Answer from the drawing. Dimensions are ordinates in mm from the lowest x, y and z of the part. Coordinates: 2 decimals unless noted, no trailing zeros. Order: outer loops, then holes, each group sorted by start corner. A loop starts at its lowest first (then second) coordinate and runs counter-clockwise, first axis right, second up. Notation, with made-up numbers: (-20, -7.75) -> (30, -7.75) arc R35 cw to (30, 31.25) -> close; hole circle Ø9 at (-14.5, 66). An arc over 180 degrees is marked (long way). Answer as a JSON object with one key per item and string values. Group by question number.
1) Consider L1, parallel to Y at x = 1.9, z = 10.5; L2, parallel to Y at x = 1.1, z = 10.75; L3, parallel to X at y = 2.2, z = 6.75. Determine where each line is inside the solid, lowest interval first.
2) Section A-A on z = 9.25 is taken. Determine the outline of the cut face in (x, y).
3) Given pin 1 (2 mm diameter, centred on x = 0.5, z = 9.5, fed in from -Y), flat-ended and moving along its own axis, determine where the tip first touches the part or whether it passes through.
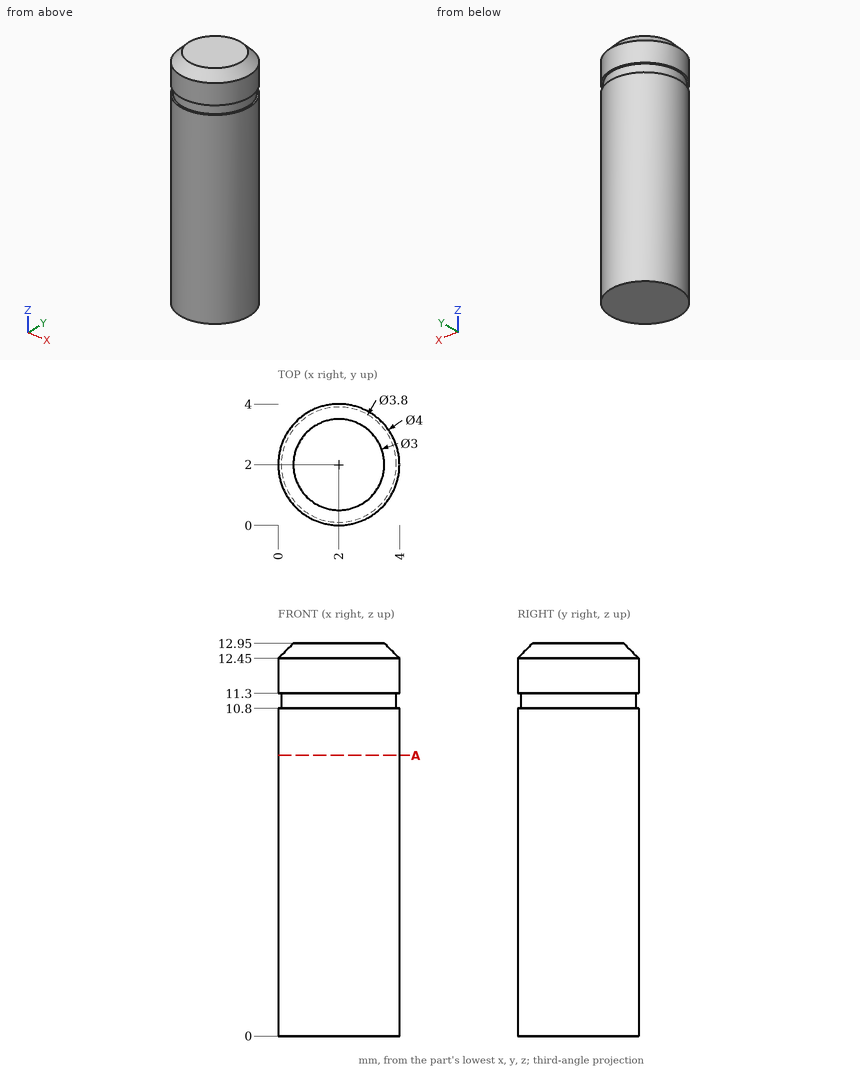
Worked answers:
{
 "1": {"L1": "y = 0 to 4", "L2": "y = 0.21 to 3.79", "L3": "x = 0.01 to 3.99"},
 "2": {"outline": "circle Ø4 at (2, 2)"},
 "3": {"pin 1": "stops at y = 0.06"}
}
